Check sheet for the modelled part. Datum: model origin and axes. Units: mm. A direction names the side the tool comes from. Give positions to 0.01 mm unless a question says otherwise; leave off trailing zeros. Write each loop counter-clockwise with the first axis right and the second up, starting at its lowest first coordinate (ties: lowest second). Pieces come first, ordered by that corner, then holes. Notation, with made-up numbers: (46.5, -32) - (61.5, -32) arc R19 cw to (61.5, -23) - close; hole circle Ø9 at (14, -5.75). An arc over 180 degrees is marked (long way). Return JSON: item names as keys, results as strings. Group by question number.
```python
from build123d import *

# Parameters (mm, degrees)
SKETCH1_R           = 63.5
BOSS_EXTRUDE1_DEPTH = 330.2
BOSS_EXTRUDE2_DEPTH = 25.4
SKETCH3_R           = 101.6
BOSS_EXTRUDE3_DEPTH = 25.4
BOSS_EXTRUDE4_DEPTH = 50.8


with BuildPart() as part:
    # Sketch1 → Boss-Extrude1 (new body)
    with BuildSketch(Plane.XY):
        Circle(SKETCH1_R)
    extrude(amount=BOSS_EXTRUDE1_DEPTH)

    # Sketch2 → Boss-Extrude2 (add)
    with BuildSketch(Plane(origin=(0, 0, 0), x_dir=(-1, 0, 0), z_dir=(0, 0, -1))):
        with BuildLine():
            Line((63.5, 0), (63.5, -254))
            ThreePointArc((63.5, -254), (0, -317.5), (-63.5, -254))
            Line((-63.5, -254), (-63.5, 0))
            ThreePointArc((-63.5, 0), (0, 63.5), (63.5, 0))
        make_face()
    extrude(amount=-BOSS_EXTRUDE2_DEPTH)

    # Sketch3 → Boss-Extrude3 (add)
    with BuildSketch(Plane.XY.offset(228.6)):
        with Locations((-19.05, 0)):
            Circle(SKETCH3_R)
    extrude(amount=-BOSS_EXTRUDE3_DEPTH)

    # Sketch5 → Boss-Extrude4 (add)
    with BuildSketch(Plane.XY.offset(203.2)):
        with BuildLine():
            Line((0, 0), (154.117737428, 111.973090562))
            ThreePointArc((154.117737428, 111.973090562), (190.5, 0), (154.117737428, -111.973090562))
            Line((154.117737428, -111.973090562), (0, 0))
        make_face()
    extrude(amount=-BOSS_EXTRUDE4_DEPTH)


solid = part.part
```
Item 1: Section check A-A on y = -80. Record the cut outline in (x, z).
Item 2: Access from +Z, -Z, +X, -X, +Y, -Y to the whole of each face (thin tool, end or side, straight path). Record for faces 1 (the face through (190.493, 1.676, 178.156)), 2 (the face through (-66, 1, 228.6)), 3 (the face through (102.03, 74.13, 178.16)), 4 (the face through (-63.5, -125, 13)), 5 (the face through (-46.8, 42.92, 100.18)).
Item 3: Section check B-B on x = 0. Record the cut outline in (y, z), plus the area to 3 significant figures.
Item 4: Section check D-D on y = -217. Record the cut outline in (x, z), plus the area to 3 significant figures.
Item 5: Section check C-C on z = 164. Record the cut outline in (x, y).
Item 6: Mould release check, pull along Z, two halves, no side actions. Record for faces 6 (the face through (-69, 1, 203.2)), 7 (the face through (-1, 1, 330.2)), 8 (the face through (63.5, -129, 13)): +Z half, -Z half, draft (parallel to the pull), parting line (faces both ways), or undercut.
Item 7: Depth check by flat-ended pin: pin 1 (4 mm diameter, centred on x = 16.5, z = 88.5, fed in from +Y); pin 2 (12.5 mm diameter, centred on y = -123.5, z = 12.5, fed in from +X); pin 3 (6 mm diameter, centred on x = -62, y = -117, fed in from +Z). Enter the tip coordinate at first touch or a pass-through.
Item 8: Material ranges on line 1 along Z through (x, y) = (22.5, -82); line 2 along Z through (x, y) = (103, 57); line 3 along X through (y, z) = (-1, 118), recorded low to high. Write a range as from..to.
Reply:
{
 "1": {"outline": "(-81.68, 203.2) - (43.58, 203.2) - (43.58, 228.6) - (-81.68, 228.6) - close; (-63.5, 0) - (63.5, 0) - (63.5, 25.4) - (-63.5, 25.4) - close; (110.11, 152.4) - (172.89, 152.4) - (172.89, 203.2) - (110.11, 203.2) - close"},
 "2": {"face 1": "+Z, -Z, +X", "face 2": "+Z", "face 3": "-Z, +Y", "face 4": "-Z, -X, +Y, -Y", "face 5": "none"},
 "3": {"outline": "(-317.5, 0) - (63.5, 0) - (63.5, 203.2) - (99.8, 203.2) - (99.8, 228.6) - (63.5, 228.6) - (63.5, 330.2) - (-63.5, 330.2) - (-63.5, 228.6) - (-99.8, 228.6) - (-99.8, 203.2) - (-63.5, 203.2) - (-63.5, 25.4) - (-317.5, 25.4) - close", "area": "50,200 mm²"},
 "4": {"outline": "(-63.5, 0) - (63.5, 0) - (63.5, 25.4) - (-63.5, 25.4) - close", "area": "3,230 mm²"},
 "5": {"outline": "(51.37, -37.32) - (154.12, -111.97) arc R190.5 ccw to (154.12, 111.97) - (51.37, 37.32) arc R63.5 ccw (long way) to start"},
 "6": {"face 6": "undercut", "face 7": "+Z half", "face 8": "draft"},
 "7": {"pin 1": "y = 61.82", "pin 2": "x = 63.5", "pin 3": "z = 25.4"},
 "8": {"line 1": "0..25.4, 203.2..228.6", "line 2": "152.4..203.2", "line 3": "-63.49..63.49"}
}
